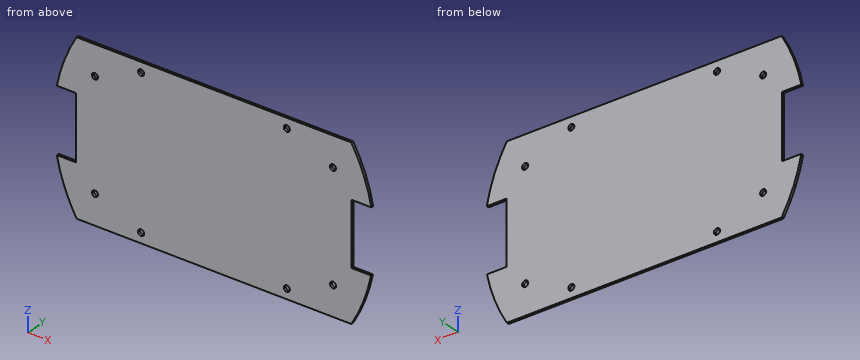
from build123d import *

# Parameters (mm, degrees)
EXTRUDE_2_DEPTH             = 1
M3X0_5_1_D                  = 2.5
M3X0_5_1_DEPTH              = 4
M3X0_5_1_TIP                = 0.751075774
M3X0_5_1_ON_FACE_2_D        = 2.5
M3X0_5_1_ON_FACE_2_DEPTH    = 4
M3X0_5_1_ON_FACE_2_TIP      = 0.751075774
PATTERN_LINEAR_1_COUNT      = 2
PATTERN_LINEAR_1_PITCH      = 98
PATTERN_LINEAR_1_COUNT_DIR2 = 2
PATTERN_LINEAR_1_PITCH_DIR2 = 44


with BuildPart() as part:
    # 草圖10 → 填料-伸長2 (new body)
    with BuildSketch(Plane(origin=(0, 0, 0), x_dir=(1, 0, 0), z_dir=(0, 1, 0))):
        with BuildLine():
            Line((56.568542495, 34), (-56.568542495, 34))
            ThreePointArc((-56.568542495, 34), (-61.540159626, 23.849711805), (-64.707032075, 13))
            Line((-64.707032075, 13), (-56.707032075, 13))
            Line((-56.707032075, 13), (-56.707032075, -12.973279994))
            Line((-56.707032075, -12.973279994), (-64.707032075, -13))
            ThreePointArc((-64.707032075, -13), (-61.540159626, -23.849711805), (-56.568542495, -34))
            Line((-56.568542495, -34), (56.568542495, -34))
            ThreePointArc((56.568542495, -34), (61.619473981, -23.644035746), (64.792427449, -12.567471713))
            Line((64.792427449, -12.567471713), (56.707032075, -12.594476939))
            Line((56.707032075, -12.594476939), (56.707032075, 13))
            Line((56.707032075, 13), (64.707032075, 13))
            ThreePointArc((64.707032075, 13), (61.540159626, 23.849711805), (56.568542495, 34))
        make_face()
    extrude(amount=EXTRUDE_2_DEPTH)

    # M3x0.5  螺絲攻的螺孔鑽1
    with Locations(Plane(origin=(30, 1, 30), x_dir=(0, 0, 1), z_dir=(0, 1, 0))):
        with Locations((0, 0), (-60, -60), (0, -60), (-60, 0)):
            Hole(M3X0_5_1_D / 2, depth=M3X0_5_1_DEPTH)
            with Locations((0, 0, -(M3X0_5_1_DEPTH + M3X0_5_1_TIP / 2))):  # 118° drill point
                Cone(0, M3X0_5_1_D / 2, M3X0_5_1_TIP, mode=Mode.SUBTRACT)

    # M3x0.5  螺絲攻的螺孔鑽1 on face 2
    with Locations(Plane(origin=(-30, 0, -30), x_dir=(0, 0, -1), z_dir=(0, -1, 0))):
        with Locations((0, 0)):
            Hole(M3X0_5_1_ON_FACE_2_D / 2, depth=M3X0_5_1_ON_FACE_2_DEPTH)
            with Locations((0, 0, -(M3X0_5_1_ON_FACE_2_DEPTH + M3X0_5_1_ON_FACE_2_TIP / 2))):  # 118° drill point
                Cone(0, M3X0_5_1_ON_FACE_2_D / 2, M3X0_5_1_ON_FACE_2_TIP, mode=Mode.SUBTRACT)

    # 草圖14 → M3x0.5  螺絲攻的螺孔鑽2 (revolve, cut)
    with BuildSketch(Plane(origin=(-49, 1, -22), x_dir=(0, 0, 1), z_dir=(1, 0, 0))):
        Polygon((0, 0), (0, 4.751075774), (1.25, 4), (1.25, 0), align=None)
    m3x0_5_2 = revolve(axis=Axis((-49, 7.35, -22), (0, -1, 0)), mode=Mode.SUBTRACT)

    # 直線複製排列1: M3x0.5 _2 2 × 2
    with Locations(*[(i * PATTERN_LINEAR_1_PITCH, 0, j * PATTERN_LINEAR_1_PITCH_DIR2) for i in range(PATTERN_LINEAR_1_COUNT) for j in range(PATTERN_LINEAR_1_COUNT_DIR2) if (i, j) != (0, 0)]):
        add(m3x0_5_2, mode=Mode.SUBTRACT)


solid = part.part
The model under review builds one solid part; all positions refer to its coordinate system, in mm. Round coordinates to 2 decimals unless told otherwise and drop trailing zeros. Loops run counter-clockwise (first coordinate to the right, second up) from the corner with the lowest first, then second, coordinate; pieces in that order, holes last. Notation, with made-up numbers: (-14, 71.25) -> (25, 71.25) arc R20 cw to (25, 78.25) -> close; hole circle Ø11 at (56, 25). An arc over 180 degrees is marked (long way). Answer as CSV lines item,"result".
1) Add section B-B on x = 49. Write out the cut boundary in (y, z).
Geometry results:
outline,"(0, -34) -> (1, -34) -> (1, -23.25) -> (0, -23.25) -> close; (0, -20.75) -> (1, -20.75) -> (1, 20.75) -> (0, 20.75) -> close; (0, 23.25) -> (1, 23.25) -> (1, 34) -> (0, 34) -> close"
2) Add section A-A on y = 0.35. State how many separate pieces and enclosed holes the cut face has, plus the area to 3 significant figures.
Geometry results:
separate pieces,"1"
enclosed holes,"8"
area,"8,060 mm²"
3) Add section D-D on z = 7. Write out the cut boundary in (x, y).
Geometry results:
outline,"(-56.71, 0) -> (56.71, 0) -> (56.71, 1) -> (-56.71, 1) -> close"
4) Add section C-C on z = -30. Write out the cut boundary in (x, y), plus the area to 3 significant figures.
Geometry results:
outline,"(-58.79, 0) -> (-31.25, 0) -> (-31.25, 1) -> (-58.79, 1) -> close; (-28.75, 0) -> (28.75, 0) -> (28.75, 1) -> (-28.75, 1) -> close; (31.25, 0) -> (58.79, 0) -> (58.79, 1) -> (31.25, 1) -> close"
area,"113 mm²"
5) To check wall thickness, follow line 1 along Z through (x, y) = (49, 0.4); line 2 along X through (y, z) = (0.5, 30); line 3 along X through (y, z) = (0.45, 21). State the ranges of each line that lie inside material, in increasing order. Write a range as from..to.
Geometry results:
line 1,"z = -34..-23.25, -20.75..20.75, 23.25..34"
line 2,"x = -58.79..-31.25, -28.75..28.75, 31.25..58.79"
line 3,"x = -62.57..-49.75, -48.25..48.25, 49.75..62.57"
